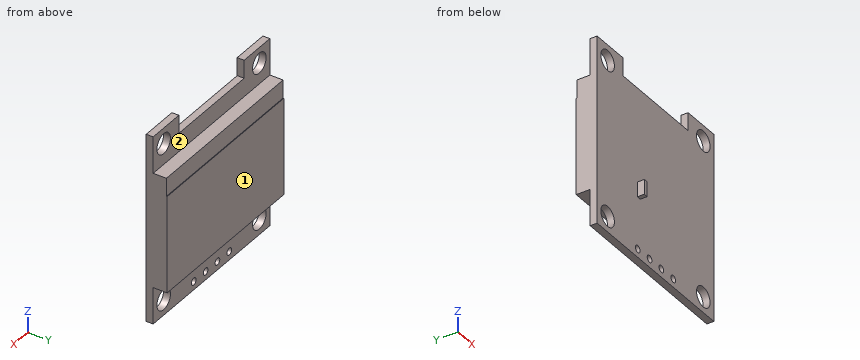
from build123d import *

# Parameters (mm, degrees)
SKETCH_1_W          = 25
SKETCH_1_H          = 27
EXTRUDE_1_DEPTH     = 1
EXTRUDE_START       = -1
SKETCH_2_W          = 25
SKETCH_2_H          = 16.5
EXTRUDE_2_DEPTH     = 2.9
EXTRUDE_START_2     = -2.9
SKETCH_3_W          = 25
SKETCH_3_H          = 13.9
EXTRUDE_3_DEPTH     = 3
SKETCH_4_W          = 14
SKETCH_4_H          = 2.6
CUT_EXTRUDE_1_DEPTH = 2
SKETCH_6_R          = 1.45
SKETCH_6_R_2        = 0.5
CUT_EXTRUDE_2_DEPTH = 2
EXTRUDE_START_3     = -3
SKETCH_7_W          = 0.62130337
SKETCH_7_H          = 2.122786517
EXTRUDE_4_DEPTH     = 4


with BuildPart() as part:
    # 草图1 → 凸台-拉伸1 (new body)
    with BuildSketch(Plane(origin=(0, 0, 0), x_dir=(1, 0, 0), z_dir=(0, 1, 0))):
        Rectangle(SKETCH_1_W, SKETCH_1_H)
    extrude(amount=EXTRUDE_1_DEPTH)

    # 草图2 → 凸台-拉伸2 (add)
    with BuildSketch(Plane(origin=(0, 1, 0), x_dir=(1, 0, 0), z_dir=(0, 1, 0)).offset(EXTRUDE_START)):
        Rectangle(SKETCH_2_W, SKETCH_2_H)
    extrude(amount=EXTRUDE_2_DEPTH)

    # 草图3 → 凸台-拉伸3 (add)
    with BuildSketch(Plane(origin=(0, 2.9, 0), x_dir=(1, 0, 0), z_dir=(0, 1, 0)).offset(EXTRUDE_START_2)):
        with Locations((0, 1.3)):
            Rectangle(SKETCH_3_W, SKETCH_3_H)
    extrude(amount=EXTRUDE_3_DEPTH)

    # 草图4 → 切除-拉伸1 (cut, through all)
    with BuildSketch(Plane(origin=(0, 1, 0), x_dir=(1, 0, 0), z_dir=(0, 1, 0))):
        with Locations((0, -12.2)):
            Rectangle(SKETCH_4_W, SKETCH_4_H)
    extrude(amount=-CUT_EXTRUDE_1_DEPTH, mode=Mode.SUBTRACT)

    # 草图6 → 切除-拉伸2 (cut, through all)
    with BuildSketch(Plane(origin=(0, 1, 0), x_dir=(1, 0, 0), z_dir=(0, 1, 0))):
        with Locations((-10.25, 11.25)):
            Circle(SKETCH_6_R)
        with Locations((10.25, 11.25)):
            Circle(SKETCH_6_R)
        with Locations((-10.25, -11.25)):
            Circle(SKETCH_6_R)
        with Locations((10.25, -11.25)):
            Circle(SKETCH_6_R)
        with Locations((-3.81, 12.3)):
            Circle(SKETCH_6_R_2)
        with Locations((-1.27, 12.3)):
            Circle(SKETCH_6_R_2)
        with Locations((1.27, 12.3)):
            Circle(SKETCH_6_R_2)
        with Locations((3.81, 12.3)):
            Circle(SKETCH_6_R_2)
    extrude(amount=-CUT_EXTRUDE_2_DEPTH, mode=Mode.SUBTRACT)

    # 草图7 → 凸台-拉伸4 (add)
    with BuildSketch(Plane.XZ.offset(EXTRUDE_START_3)):
        with Locations((-3.572494382, -3.753707866)):
            Rectangle(SKETCH_7_W, SKETCH_7_H)
    extrude(amount=EXTRUDE_4_DEPTH)


solid = part.part
CAD build for the part. Positions are in the model's coordinates, mm. Face numbers are marked on the shaded views. A direction names the side the tool comes from. Round coordinates to 2 decimals unless told otherwise and drop trailing zeros. Write each loop counter-clockwise with the first axis right and the second up, starting at its lowest first coordinate (ties: lowest second). Pieces come first, ordered by that corner, then holes. Notation, with made-up numbers: M 17.25,38.25 L 64.25,38.25 A26 cw 64.25,57.25 Z; hole C 43,35 d9. An arc over 180 degrees is marked long. Put each result on its own line as item: value. Start each with the question number.
1) Saw through at B-B, the plane z = -11.25. Write the cut outline in (x, y), and give its area (3 significant figures).
2) Saw through at C-C, the plane y = 0.5. Count the separate pieces of the cut face and the enclosed holes in it, and give its area (3 significant figures).
3) Drill centre lines: probe 1 along X at (y, z) = (0.3, -11.25); probe 2 along X at (y, z) = (0.2, 11.25); probe 3 along Z at (x, y) = (-3.81, 0.3). Where is each one in solid material? Low to high. Write a range as [from, to].
4) 3-axis set-ups, long thin cutter, end or side, ignore diameter. For the marked faces 1 and 2: which of +Z, -Z, +X, -X, +Y, -Y reach the whole face in a straight line?
5) Saw through at D-D, the plane x = 1.27. Write the cut outline in (y, z).
6) Pin check, flat tips, straight feed: pin 1 Ø1 at (x, y) = (-3, 2) entering from -Z; pin 2 Ø0.7 at (x, y) = (-3.5, -0.5) entering from -Z; pin 3 Ø1.1 at (y, z) = (-0.5, -3.5) entering from +X; pin 4 Ø2.5 at (x, z) = (1.5, 11.5) entering from +Y. Stop position of each tip, or through.
7) Saw through at A-A, the plane x = 10.25. Write the cut outline in (y, z).
Resolved:
1. outline: M -12.5,0 L -11.7,0 L -11.7,1 L -12.5,1 Z; M -8.8,0 L 8.8,0 L 8.8,1 L -8.8,1 Z; M 11.7,0 L 12.5,0 L 12.5,1 L 11.7,1 Z
1. area: 19.2 mm²
2. separate pieces: 1
2. enclosed holes: 8
2. area: 609 mm²
3. probe 1: [-12.5, -11.7], [-8.8, 8.8], [11.7, 12.5]
3. probe 2: [-12.5, -11.7], [-8.8, -7], [7, 8.8], [11.7, 12.5]
3. probe 3: [-13.5, -12.8], [-11.8, 10.9]
4. face 1: +Z, -Z, +X, -X, +Y
4. face 2: +Z, +X, -X, +Y
5. outline: M 0,-13.5 L 1,-13.5 L 1,-12.8 L 0,-12.8 Z; M 0,-11.8 L 1,-11.8 L 1,-8.25 L 3,-8.25 L 3,5.65 L 2.9,5.65 L 2.9,8.25 L 1,8.25 L 1,10.9 L 0,10.9 Z
6. pin 1: z = -8.25
6. pin 2: z = -4.82
6. pin 3: x = 12.5
6. pin 4: y = 1
7. outline: M 0,-13.5 L 1,-13.5 L 1,-12.7 L 0,-12.7 Z; M 0,-9.8 L 1,-9.8 L 1,-8.25 L 3,-8.25 L 3,5.65 L 2.9,5.65 L 2.9,8.25 L 1,8.25 L 1,9.8 L 0,9.8 Z; M 0,12.7 L 1,12.7 L 1,13.5 L 0,13.5 Z
